Can you work these out from the model? Positions are in its coordinate system, mm. A direction names the side the tool comes from. Give positions to 0.01 mm unless a question says otherwise; leave off trailing zeros. Write each loop counter-clockwise with the first axis right and the second up, starting at its lowest first coordinate (ties: lowest second). Pieces come first, ordered by that corner, then holes.
```python
from build123d import *

# Parameters (mm, degrees)
BOSS_EXTRUDE1_DEPTH = 3
BOSS_EXTRUDE2_DEPTH = 20
SKETCH3_R           = 3.5
CUT_EXTRUDE1_DEPTH  = 20
BOSS_EXTRUDE3_DEPTH = 3
FILLET1_R           = 10
FILLET3_R           = 5
BOSS_EXTRUDE4_DEPTH = 20
CUT_EXTRUDE2_DEPTH  = 20
CUT_EXTRUDE4_DEPTH  = 20


with BuildPart() as part:
    # Sketch1 → Boss-Extrude1 (new body)
    with BuildSketch(Plane.XY):
        with BuildLine():
            Line((-35, 10), (24.289684969, 10))
            ThreePointArc((24.289684969, 10), (37.289684969, -3), (24.289684969, -16))
            Line((24.289684969, -16), (-35, -16))
            Line((-35, -16), (-35, 10))
        make_face()
    extrude(amount=-BOSS_EXTRUDE1_DEPTH)

    # Sketch2 → Boss-Extrude2 (add)
    with BuildSketch(Plane(origin=(0, 0, -3), x_dir=(-1, 0, 0), z_dir=(0, 0, -1))):
        with BuildLine():
            Line((-24.289684969, 7), (35, 7))
            Line((35, 7), (35, 10))
            Line((35, 10), (-24.289684969, 10))
            ThreePointArc((-24.289684969, 10), (-37.289684969, -3), (-24.289684969, -16))
            Line((-24.289684969, -16), (35, -16))
            Line((35, -16), (35, -13))
            Line((35, -13), (-24.289684969, -13))
            ThreePointArc((-24.289684969, -13), (-34.289684969, -3), (-24.289684969, 7))
        make_face()
    extrude(amount=BOSS_EXTRUDE2_DEPTH)

    # Sketch3 → Cut-Extrude1 (cut)
    with BuildSketch(Plane.XY):
        with Locations((24.289684969, -3)):
            Circle(SKETCH3_R)
    extrude(amount=-CUT_EXTRUDE1_DEPTH, mode=Mode.SUBTRACT)

    # Sketch4 → Boss-Extrude3 (add)
    with BuildSketch(Plane.XY):
        with BuildLine():
            Line((24.289684969, -16), (-35, -16))
            Line((-35, -16), (-35, -90))
            Line((-35, -90), (15, -90))
            Line((15, -90), (36.86764108, -6.285577584))
            ThreePointArc((36.86764108, -6.285577584), (32.235988871, -13.288646864), (24.289684969, -16))
        make_face()
    extrude(amount=-BOSS_EXTRUDE3_DEPTH)

    # Fillet1
    fillet1_edges = [part.edges().sort_by_distance(p)[0] for p in [
        (15, -90, -1.5),
    ]]
    fillet(fillet1_edges, radius=FILLET1_R)

    # Fillet3
    fillet3_edges = [part.edges().sort_by_distance(p)[0] for p in [
        (-35, -90, -1.5),
    ]]
    fillet(fillet3_edges, radius=FILLET3_R)

    # Sketch5 → Boss-Extrude4 (add)
    with BuildSketch(Plane(origin=(0, 0, -3), x_dir=(-1, 0, 0), z_dir=(0, 0, -1))):
        with BuildLine():
            Line((-14.049374385, -81.769157161), (-31.865646811, -13.564317402))
            ThreePointArc((-31.865646811, -13.564317402), (-35.003699882, -10.362736207), (-36.86764108, -6.285577584))
            Line((-36.86764108, -6.285577584), (-16.951979641, -82.527367373))
            ThreePointArc((-16.951979641, -82.527367373), (-13.389170249, -87.914343742), (-7.276628786, -90))
            Line((-7.276628786, -90), (30, -90))
            Line((30, -90), (30, -87))
            Line((30, -87), (-7.276628786, -87))
            ThreePointArc((-7.276628786, -87), (-11.55540781, -85.540040619), (-14.049374385, -81.769157161))
        make_face()
    extrude(amount=BOSS_EXTRUDE4_DEPTH)

    # Sketch7 → Cut-Extrude2 (cut)
    with BuildSketch(Plane(origin=(0, 0, -3), x_dir=(-1, 0, 0), z_dir=(0, 0, -1))):
        with BuildLine():
            ThreePointArc((-2.5, -3), (0, -5.5), (2.5, -3))
            Line((2.5, -3), (-2.5, -3))
        make_face()
        with BuildLine():
            Line((-2.5, -3), (2.5, -3))
            ThreePointArc((2.5, -3), (0, -0.5), (-2.5, -3))
        make_face()
        with BuildLine():
            ThreePointArc((17.5, -3), (20, -5.5), (22.5, -3))
            Line((22.5, -3), (17.5, -3))
        make_face()
        with BuildLine():
            Line((17.5, -3), (22.5, -3))
            ThreePointArc((22.5, -3), (20, -0.5), (17.5, -3))
        make_face()
    extrude(amount=-CUT_EXTRUDE2_DEPTH, mode=Mode.SUBTRACT)

    # Sketch6 → Cut-Extrude4 (cut)
    with BuildSketch(Plane(origin=(0, 0, -3), x_dir=(-1, 0, 0), z_dir=(0, 0, -1))):
        with BuildLine():
            Line((20.361685607, -56), (20.361685607, -47))
            ThreePointArc((20.361685607, -47), (11.361685607, -38), (2.361685607, -47))
            Line((2.361685607, -47), (2.361685607, -56))
            ThreePointArc((2.361685607, -56), (11.361685607, -65), (20.361685607, -56))
        make_face()
    extrude(amount=-CUT_EXTRUDE4_DEPTH, mode=Mode.SUBTRACT)


solid = part.part
```
1) For pin 1 Ø8 at (x, y) = (-20, -3) entering from +Z; pin 2 Ø8 at (x, y) = (19.5, -31) entering from -Z; pin 3 Ø2 at (y, z) = (-19, -5.5) entering from -X; pin 4 Ø2.5 at (y, z) = (-51, -2) entering from +X, each with a flat end and sliding along its axis, tell me the tip position at first contact or that it passes through.
Values follow:
pin 1: stops at z = 0
pin 2: stops at z = -3
pin 3: stops at x = 30.18
pin 4: stops at x = 25.51
2) Suppose I cut it at D-D on z = -9.75. Write out the boundary of the cut face in (x, y).
Values follow:
outline: (-35, -16) - (24.29, -16) arc R13 ccw to (31.87, -13.56) - (14.05, -81.77) arc R7 cw to (7.28, -87) - (-30, -87) - (-30, -90) - (7.28, -90) arc R10 ccw to (16.95, -82.53) - (36.87, -6.29) arc R13 ccw to (24.29, 10) - (-35, 10) - (-35, 7) - (24.29, 7) arc R10 cw to (24.29, -13) - (-35, -13) - close
3) If we mould it in two halves opening along Y, with no side actions, what happens to faces 1 (the face through (27.05, -43.87, -11.34)), 2 (the face through (34.476, 5.077, -11.339)), 3 (the face through (22.833, -48.144, -12.86))? For each: +Y half, -Y half, draft (parallel to the pull), parting line (faces both ways), or undercut.
Values follow:
face 1: -Y half
face 2: parting line
face 3: undercut
4) For faces 4 (the face through (-2.362, -51, -2)), 5 (the face through (-11, -90, -11)), 6 (the face through (0, 2, -3)), which set-ups out of +Z, -Z, +X, -X, +Y, -Y let a thin tool reach every point of the face, with its end or its side?
Values follow:
face 4: +Z, -Z
face 5: +Z, -Z, +X, -X, -Y
face 6: -Z, -X
5) Suppose I cut it at C-C on y = -40.5. Write out the boundary of the cut face in (x, z), plus the area to 3 significant figures.
Values follow:
outline: (-35, -3) - (-17.59, -3) - (-17.59, 0) - (-35, 0) - close; (-5.14, -3) - (24.83, -3) - (24.83, -23) - (27.93, -23) - (27.93, 0) - (-5.14, 0) - close
area: 213 mm2
6) Suppose I cut it at B-B on x = 0. Write out the boundary of the cut face in (y, z).
Values follow:
outline: (-90, -23) - (-87, -23) - (-87, -3) - (-16, -3) - (-16, -23) - (-13, -23) - (-13, -3) - (-5.5, -3) - (-5.5, 0) - (-90, 0) - close; (-0.5, -3) - (7, -3) - (7, -23) - (10, -23) - (10, 0) - (-0.5, 0) - close
7) Please list where these lines run through material, in increasing order: L1, parallel to Y at x = -24.5, z = -19.75; L2, parallel to Y at x = 0, z = -1.05; L3, parallel to Y at x = 13, z = -15.
Values follow:
L1: y = -90 to -87, -16 to -13, 7 to 10
L2: y = -90 to -5.5, -0.5 to 10
L3: y = -88.2 to -84.03, -16 to -13, 7 to 10
8) Suppose I cut it at A-A on y = -3. Write out the boundary of the cut face in (x, z).
Values follow:
outline: (-35, -3) - (-22.5, -3) - (-22.5, 0) - (-35, 0) - close; (-17.5, -3) - (-2.5, -3) - (-2.5, 0) - (-17.5, 0) - close; (2.5, -3) - (20.79, -3) - (20.79, 0) - (2.5, 0) - close; (27.79, -3) - (34.29, -3) - (34.29, -23) - (37.29, -23) - (37.29, 0) - (27.79, 0) - close
